Print and shaded views of the part. All mm, measured from the part's lowest x, y and z. A direction names the side the tool comes from. Coordinates: 2 decimals unless noted, no trailing zeros. Order: outer loops, then holes, each group sorted by start corner. A loop starts at its lowest first (then second) coordinate and runs counter-clockwise, first axis right, second up. Notation, with made-up numbers: M 11,45 L 37,45 A15 cw 37,61 Z; hole C 14.25,43.25 d2. An arc over 180 degrees is marked long. Use a Markdown table: item, result. Add a question column.
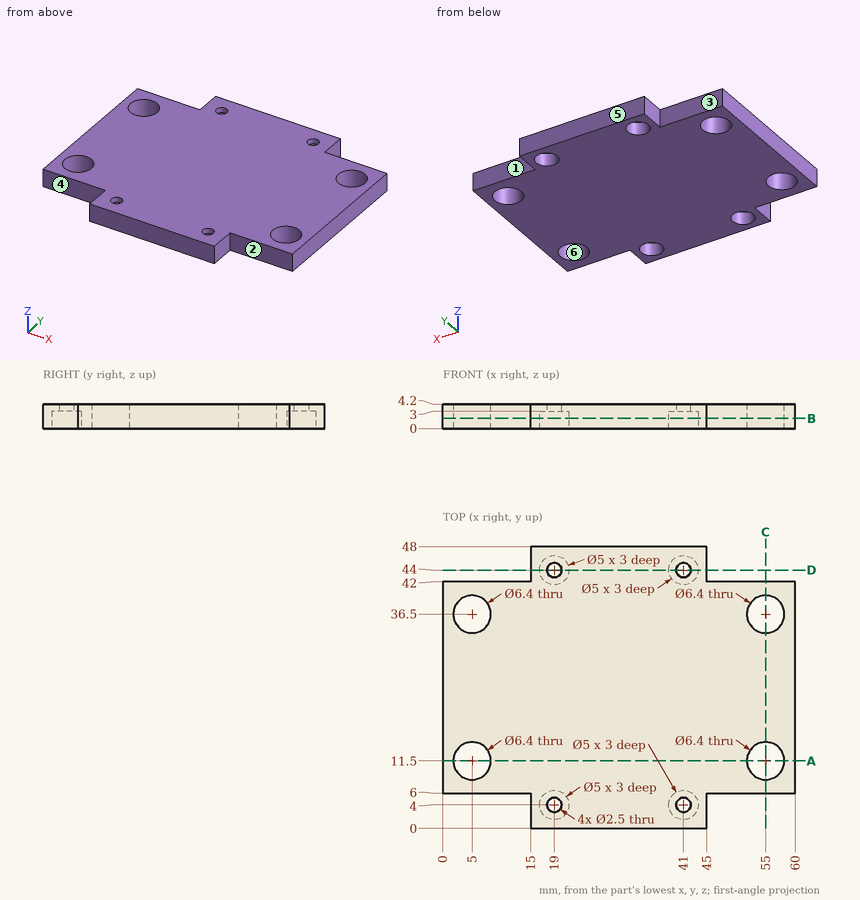
(1) Slice it at D-D on y = 44. Give the cut face in (x, z).
(2) Slice it at A-A on y = 11.5. Give the cut face in (x, z).
(3) Drop flat-ended pins along their axis: P1, Ø3, axis at x = 19, y = 44, coming from the -Z side; P2, Ø4, axis at x = 41, y = 44, coming from the +Z side; P3, Ø5, axis at x = 55, y = 36.5, coming from the +Z side; P4, Ø1.3, axis at y = 46, z = 1, coming from the +X side. Give the stop position or say it passes through.
(4) Slice it at C-C on x = 55. Give the cut face in (y, z), and give its area (3 significant figures).
(5) Which spindle directions (+Z, -Z, +X, -X, +Y, -Y) get a long thin tool onto all of the face, cutting with end or side? Do the marked faces 1, 2 and 3. Say none if no direction does.
(6) Mould opens along Y. For the marked faces 4, 5 and 6 say: released by +Y, released by -Y, zero draft, split by the parting line, or undercut.
(7) Slice it at B-B on z = 1.75. State how many separate pieces and enclosed holes the cut face has, and give its area (3 significant figures).
(8) Drill centre lines: line 1 along Y through (x, z) = (19, 3.6); line 2 along X through (y, z) = (4, 3.65); line 3 along X through (y, z) = (45.5, 0.3). Where is each one in solid material? Low to high. Write a range as from..to.
Solutions:
| question | item | result |
|---|---|---|
| 1 | outline | M 15,0 L 16.5,0 L 16.5,3 L 17.75,3 L 17.75,4.2 L 15,4.2 Z; M 20.25,3 L 21.5,3 L 21.5,0 L 38.5,0 L 38.5,3 L 39.75,3 L 39.75,4.2 L 20.25,4.2 Z; M 42.25,3 L 43.5,3 L 43.5,0 L 45,0 L 45,4.2 L 42.25,4.2 Z |
| 2 | outline | M 0,0 L 1.8,0 L 1.8,4.2 L 0,4.2 Z; M 8.2,0 L 51.8,0 L 51.8,4.2 L 8.2,4.2 Z; M 58.2,0 L 60,0 L 60,4.2 L 58.2,4.2 Z |
| 3 | P1 | z = 3 |
| 3 | P2 | z = 4.2 |
| 3 | P3 | through |
| 3 | P4 | x = 45 |
| 4 | outline | M 6,0 L 8.3,0 L 8.3,4.2 L 6,4.2 Z; M 14.7,0 L 33.3,0 L 33.3,4.2 L 14.7,4.2 Z; M 39.7,0 L 42,0 L 42,4.2 L 39.7,4.2 Z |
| 4 | area | 97.4 mm² |
| 5 | face 1 | +Z, -Z, +X, +Y |
| 5 | face 2 | +Z, -Z, +X, -Y |
| 5 | face 3 | +Z, -Z, -X, +Y |
| 6 | face 4 | released by -Y |
| 6 | face 5 | released by +Y |
| 6 | face 6 | undercut |
| 7 | separate pieces | 1 |
| 7 | enclosed holes | 8 |
| 7 | area | 2,310 mm² |
| 8 | line 1 | 0..2.75, 5.25..42.75, 45.25..48 |
| 8 | line 2 | 15..17.75, 20.25..39.75, 42.25..45 |
| 8 | line 3 | 15..17, 21..39, 43..45 |
